Source: CAD feature listing. Evaluate the final solid. Frame: model axes, mm. A direction names the side the tool comes from. Give positions to 0.01 mm unless a question says otherwise; leave off trailing zeros. Order: outer loops, then holes, each group sorted by start corner. A loop starts at its lowest first (then second) coordinate and runs counter-clockwise, first axis right, second up.
```python
from build123d import *

# Parameters (mm, degrees)
EXTRUDE_1_DEPTH     = 240
SKETCH_2_R          = 1
CUT_EXTRUDE_1_DEPTH = 10
CHAMFER_1_SIZE      = 0.5
SKETCH_3_R          = 2.383304988
CUT_EXTRUDE_2_DEPTH = 1


with BuildPart() as part:
    # 草图1 → 凸台-拉伸1 (new body)
    with BuildSketch(Plane(origin=(0, 0, 0), x_dir=(1, 0, 0), z_dir=(0, 1, 0))):
        Polygon((-3.5, 0.4), (-3.5, -2.4), (3.5, -2.4), (3.5, 0.4), (2.5, 0.4), (2.5, 1.4), (3.5, 1.4), (3.5, 2.4), (-3.5, 2.4), (-3.5, 1.4), (-2.5, 1.4), (-2.5, 0.4), align=None)
    extrude(amount=EXTRUDE_1_DEPTH)

    # 草图2 → 切除-拉伸1 (cut)
    with BuildSketch(Plane(origin=(0, 0, -2.4), x_dir=(-1, 0, 0), z_dir=(0, 0, -1))):
        with Locations((0, 5)):
            Circle(SKETCH_2_R)
        with Locations((0, 20)):
            Circle(SKETCH_2_R)
        with Locations((0, 35)):
            Circle(SKETCH_2_R)
        with Locations((0, 50)):
            Circle(SKETCH_2_R)
        with Locations((0, 65)):
            Circle(SKETCH_2_R)
        with Locations((0, 80)):
            Circle(SKETCH_2_R)
        with Locations((0, 95)):
            Circle(SKETCH_2_R)
        with Locations((0, 110)):
            Circle(SKETCH_2_R)
        with Locations((0, 125)):
            Circle(SKETCH_2_R)
        with Locations((0, 140)):
            Circle(SKETCH_2_R)
        with Locations((0, 155)):
            Circle(SKETCH_2_R)
        with Locations((0, 170)):
            Circle(SKETCH_2_R)
        with Locations((0, 185)):
            Circle(SKETCH_2_R)
        with Locations((0, 200)):
            Circle(SKETCH_2_R)
        with Locations((0, 215)):
            Circle(SKETCH_2_R)
        with Locations((0, 230)):
            Circle(SKETCH_2_R)
    extrude(amount=-CUT_EXTRUDE_1_DEPTH, mode=Mode.SUBTRACT)

    # 倒角1
    chamfer_1_edges = [part.edges().sort_by_distance(p)[0] for p in [
        (-3.5, 120, -2.4),
        (3.5, 120, -2.4),
        (3.5, 120, 2.4),
        (-3.5, 120, 2.4),
    ]]
    chamfer(chamfer_1_edges, length=CHAMFER_1_SIZE)

    # 草图3 → 切除-拉伸2 (cut)
    with BuildSketch(Plane(origin=(0, 0, -2.4), x_dir=(-1, 0, 0), z_dir=(0, 0, -1))):
        with Locations((0, 5)):
            Circle(SKETCH_3_R)
        with Locations((0, 20)):
            Circle(SKETCH_3_R)
        with Locations((0, 35)):
            Circle(SKETCH_3_R)
        with Locations((0, 50)):
            Circle(SKETCH_3_R)
        with Locations((0, 65)):
            Circle(SKETCH_3_R)
        with Locations((0, 80)):
            Circle(SKETCH_3_R)
        with Locations((0, 95)):
            Circle(SKETCH_3_R)
        with Locations((0, 110)):
            Circle(SKETCH_3_R)
        with Locations((0, 125)):
            Circle(SKETCH_3_R)
        with Locations((0, 140)):
            Circle(SKETCH_3_R)
        with Locations((0, 155)):
            Circle(SKETCH_3_R)
        with Locations((0, 170)):
            Circle(SKETCH_3_R)
        with Locations((0, 185)):
            Circle(SKETCH_3_R)
        with Locations((0, 200)):
            Circle(SKETCH_3_R)
        with Locations((0, 215)):
            Circle(SKETCH_3_R)
        with Locations((0, 230)):
            Circle(SKETCH_3_R)
    extrude(amount=-CUT_EXTRUDE_2_DEPTH, mode=Mode.SUBTRACT)


solid = part.part
```
1) Material intervals for L1, parallel to Z at x = 3, y = 210; L2, parallel to Z at x = -1.5, y = 214.5; L3, parallel to X at y = 200, z = -1.8, sorted ascending.
Report:
L1: z = -2.4 to -1.4, -0.4 to 2.4
L2: z = -1.4 to 2.4
L3: x = -3.5 to -2.38, 2.38 to 3.5
2) Reachability of faces 3 (the cylindrical face through (0.517, 92.673, -1.907)), 4 (the flat face through (0, 0, 0)) from +Z, -Z, +X, -X, +Y, -Y: full face, straight path, thin tool, end or side. Return the list, or none.
Report:
face 3: -Z
face 4: +Z, -Z, +X, -X, -Y
3) Pin query (flat end, axial travel): pin 1 (4 mm diameter, centred on x = 0, y = 50, fed in from +Z); pin 2 (2.5 mm diameter, centred on x = 0, y = 50, fed in from -Z). Return the tip coordinate at first contact, or that it passes through.
Report:
pin 1: stops at z = 2.4
pin 2: stops at z = -1.4
4) Section query A-A, the plane z = 0.4. Count the separate pieces of the cut face and the enclosed holes in it, and give its area (3 significant figures).
Report:
separate pieces: 1
enclosed holes: 16
area: 1,630 mm2
5) Draft query along X for faces 1 (the cylindrical face through (0.517, 107.673, -1.907)), 2 (the flat face through (0, 240, 0)). Return one class per face: +X half, -X half, draft (parallel to the pull), parting line (faces both ways), or undercut.
Report:
face 1: undercut
face 2: draft
6) Section query B-B, the plane y = 24.5. Return the cut outline in (x, z).
Report:
outline: (-3.5, -1.9) - (-3, -2.4) - (3, -2.4) - (3.5, -1.9) - (3.5, -1.4) - (2.5, -1.4) - (2.5, -0.4) - (3.5, -0.4) - (3.5, 1.9) - (3, 2.4) - (-3, 2.4) - (-3.5, 1.9) - (-3.5, -0.4) - (-2.5, -0.4) - (-2.5, -1.4) - (-3.5, -1.4) - close
